CAD build for the part. Positions are in the model's coordinates, mm. Face numbers are marked on the shaded views. Round coordinates to 2 decimals unless told otherwise and drop trailing zeros. Write each loop counter-clockwise with the first axis right and the second up, starting at its lowest first coordinate (ties: lowest second). Pieces come first, ordered by that corner, then holes. Notation, with made-up numbers: (43.25, 20) -> (60.25, 20) arc R18 ccw to (60.25, 34) -> close; hole circle Ø7 at (10.5, -4.75). An arc over 180 degrees is marked (long way). Put each result on its own line as item: value. Start each with the question number.
1. Saw through at D-D on y = 2.75. List the corners of the cut face in (x, z).
2. Pull direction Z, two halves, no side cores. Call the marked faces 1, 2 and 3: pulls with the +Z half, pulls with the -Z half, needs draft (parallel to the pull), parting line crosses it, or undercut.
3. Saw through at C-C on z = -6.5. List the corners of the cut face in (x, y), and give its area (3 significant figures).
4. Saw through at A-A on x = 11. List the corners of the cut face in (y, z).
5. Drill centre lines: line 1 (Z direction, x = -7.5, y = 3.5); line 2 (X direction, y = 2.5, z = 4); line 3 (Z direction, x = 14.5, y = 1.5). Where is each one in solid material? Low to high. Write a range as from..to.
6. Flat gauge pins, fed straight in: P1, Ø1.9, axis at x = 27.81, y = 9.83, coming from the +Z side; P2, Ø8, axis at x = -13, y = 13.5, coming from the -Z side; P3, Ø5, axis at y = 7, z = -2.5, coming from the +X side; P4, Ø6, axis at x = -3, z = -7.5, coming from the +Y side. Where does each tip first touch, or does it go through?
7. Saw through at B-B on z = 3.5. List the corners of the cut face in (x, y).
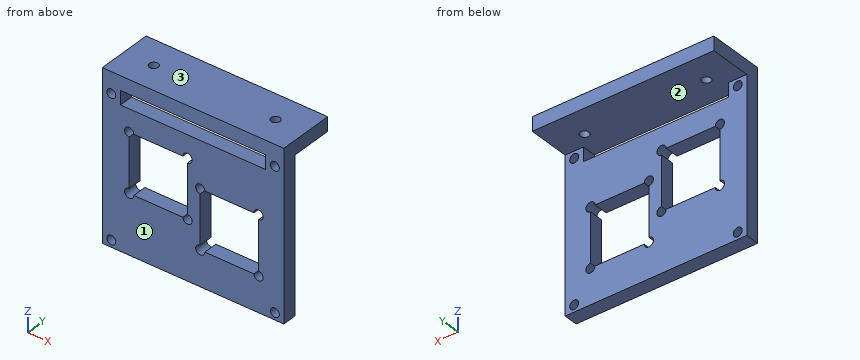
from build123d import *

# Parameters (mm, degrees)
SKETCH_1_R          = 1.6
EXTRUDE_1_DEPTH     = 5
SKETCH_2_R          = 1.65
SKETCH_2_W          = 20.88
SKETCH_2_H          = 20.88
CUT_EXTRUDE_1_DEPTH = 5
SKETCH_4_W          = 65
SKETCH_4_H          = 5
EXTRUDE_2_DEPTH     = 5
SKETCH_5_W          = 65
SKETCH_5_H          = 5
EXTRUDE_3_DEPTH     = 15
SKETCH_6_R          = 1.6
CUT_EXTRUDE_2_DEPTH = 15


with BuildPart() as part:
    # 草图1 → 凸台-拉伸1 (new body)
    with BuildSketch(Plane(origin=(0, 0, 0), x_dir=(1, 0, 0), z_dir=(0, 1, 0))):
        Polygon((-19.989784722, -25.876557595), (32.010215278, -25.876557595), (32.010215278, -30.876557595), (38.510215278, -30.876557595), (38.510215278, 24.123442405), (-26.489784722, 24.123442405), (-26.489784722, -30.876557595), (-19.989784722, -30.876557595), align=None)
        with Locations(Location((-23.259784722, 21.623442405, 0), (0, 0, 270))):
            Circle(SKETCH_1_R, mode=Mode.SUBTRACT)
        with Locations(Location((-23.259784722, -28.376557595, 0), (0, 0, 270))):
            Circle(SKETCH_1_R, mode=Mode.SUBTRACT)
        with Locations(Location((35.280215278, -28.376557595, 0), (0, 0, 270))):
            Circle(SKETCH_1_R, mode=Mode.SUBTRACT)
        with Locations(Location((35.280215278, 21.623442405, 0), (0, 0, 270))):
            Circle(SKETCH_1_R, mode=Mode.SUBTRACT)
    extrude(amount=EXTRUDE_1_DEPTH)

    # 草图2 → 切除-拉伸1 (cut)
    with BuildSketch(Plane(origin=(0, 5, 0), x_dir=(1, 0, 0), z_dir=(0, 1, 0))):
        with BuildLine():
            ThreePointArc((5.678835194, 2.978753935), (4.028835194, 4.628753935), (2.378835194, 2.978753935))
            Line((2.378835194, 2.978753935), (4.028835194, 2.978753935))
            Line((4.028835194, 2.978753935), (4.028835194, 1.328753935))
            ThreePointArc((4.028835194, 1.328753935), (5.195561383, 1.812027746), (5.678835194, 2.978753935))
        make_face()
        with BuildLine():
            Line((4.028835194, 2.978753935), (2.378835194, 2.978753935))
            ThreePointArc((2.378835194, 2.978753935), (2.862109005, 1.812027746), (4.028835194, 1.328753935))
            Line((4.028835194, 1.328753935), (4.028835194, 2.978753935))
        make_face()
        with Locations((-16.851164806, -17.901246065)):
            Circle(SKETCH_2_R)
        with Locations((4.028835194, -17.901246065)):
            Circle(SKETCH_2_R)
        with Locations((4.028835194, 2.978753935)):
            Circle(SKETCH_2_R)
        with Locations((-16.851164806, 2.978753935)):
            Circle(SKETCH_2_R)
        with Locations((-6.411164806, -7.461246065)):
            Rectangle(SKETCH_2_W, SKETCH_2_H)
        with BuildLine():
            ThreePointArc((5.678835194, -17.901246065), (5.195561383, -16.734519876), (4.028835194, -16.251246065))
            Line((4.028835194, -16.251246065), (4.028835194, -17.901246065))
            Line((4.028835194, -17.901246065), (2.378835194, -17.901246065))
            ThreePointArc((2.378835194, -17.901246065), (4.028835194, -19.551246065), (5.678835194, -17.901246065))
        make_face()
        with BuildLine():
            Line((4.028835194, -17.901246065), (4.028835194, -16.251246065))
            ThreePointArc((4.028835194, -16.251246065), (2.862109005, -16.734519876), (2.378835194, -17.901246065))
            Line((2.378835194, -17.901246065), (4.028835194, -17.901246065))
        make_face()
        with BuildLine():
            ThreePointArc((-15.201164806, -17.901246065), (-15.684438617, -16.734519876), (-16.851164806, -16.251246065))
            Line((-16.851164806, -16.251246065), (-16.851164806, -17.901246065))
            Line((-16.851164806, -17.901246065), (-15.201164806, -17.901246065))
        make_face()
        with BuildLine():
            Line((-16.851164806, -17.901246065), (-16.851164806, -16.251246065))
            ThreePointArc((-16.851164806, -16.251246065), (-18.017890995, -19.067972254), (-15.201164806, -17.901246065))
            Line((-15.201164806, -17.901246065), (-16.851164806, -17.901246065))
        make_face()
        with BuildLine():
            ThreePointArc((10.220215278, -9.316557595), (9.736941467, -8.149831407), (8.570215278, -7.666557595))
            Line((8.570215278, -7.666557595), (8.570215278, -9.316557595))
            Line((8.570215278, -9.316557595), (10.220215278, -9.316557595))
        make_face()
        with BuildLine():
            Line((8.570215278, -9.316557595), (8.570215278, -7.666557595))
            ThreePointArc((8.570215278, -7.666557595), (7.403489089, -10.483283784), (10.220215278, -9.316557595))
            Line((10.220215278, -9.316557595), (8.570215278, -9.316557595))
        make_face()
        with Locations((8.570215278, -9.316557595)):
            Circle(SKETCH_2_R)
        with Locations((29.450215278, -9.316557595)):
            Circle(SKETCH_2_R)
        with Locations((29.450215278, 11.563442405)):
            Circle(SKETCH_2_R)
        with Locations((8.570215278, 11.563442405)):
            Circle(SKETCH_2_R)
        with Locations((19.010215278, 1.123442405)):
            Rectangle(SKETCH_2_W, SKETCH_2_H)
        with BuildLine():
            ThreePointArc((31.100215278, 11.563442405), (29.450215278, 13.213442405), (27.800215278, 11.563442405))
            Line((27.800215278, 11.563442405), (29.450215278, 11.563442405))
            Line((29.450215278, 11.563442405), (29.450215278, 9.913442405))
            ThreePointArc((29.450215278, 9.913442405), (30.616941467, 10.396716216), (31.100215278, 11.563442405))
        make_face()
        with BuildLine():
            Line((29.450215278, 11.563442405), (27.800215278, 11.563442405))
            ThreePointArc((27.800215278, 11.563442405), (28.283489089, 10.396716216), (29.450215278, 9.913442405))
            Line((29.450215278, 9.913442405), (29.450215278, 11.563442405))
        make_face()
        with BuildLine():
            ThreePointArc((31.100215278, -9.316557595), (30.616941467, -8.149831407), (29.450215278, -7.666557595))
            Line((29.450215278, -7.666557595), (29.450215278, -9.316557595))
            Line((29.450215278, -9.316557595), (27.800215278, -9.316557595))
            ThreePointArc((27.800215278, -9.316557595), (29.450215278, -10.966557595), (31.100215278, -9.316557595))
        make_face()
        with BuildLine():
            Line((29.450215278, -9.316557595), (29.450215278, -7.666557595))
            ThreePointArc((29.450215278, -7.666557595), (28.283489089, -8.149831407), (27.800215278, -9.316557595))
            Line((27.800215278, -9.316557595), (29.450215278, -9.316557595))
        make_face()
    extrude(amount=-CUT_EXTRUDE_1_DEPTH, mode=Mode.SUBTRACT)

    # 草图4 → 凸台-拉伸2 (add)
    with BuildSketch(Plane.XY.offset(30.876557595)):
        with Locations((6.010215278, 2.5)):
            Rectangle(SKETCH_4_W, SKETCH_4_H)
    extrude(amount=EXTRUDE_2_DEPTH)

    # 草图5 → 凸台-拉伸3 (add)
    with BuildSketch(Plane(origin=(0, 5, 0), x_dir=(1, 0, 0), z_dir=(0, 1, 0))):
        with Locations((6.010215278, -33.376557595)):
            Rectangle(SKETCH_5_W, SKETCH_5_H)
    extrude(amount=EXTRUDE_3_DEPTH)

    # 草图6 → 切除-拉伸2 (cut)
    with BuildSketch(Plane(origin=(0, 0, 30.876557595), x_dir=(-1, 0, 0), z_dir=(0, 0, -1))):
        with Locations((-27.810215278, 9.832763387)):
            Circle(SKETCH_6_R)
        with Locations((15.789784722, 9.832763387)):
            Circle(SKETCH_6_R)
    extrude(amount=-CUT_EXTRUDE_2_DEPTH, mode=Mode.SUBTRACT)


solid = part.part
Return value:
1. outline: (-26.49, -24.12) -> (38.51, -24.12) -> (38.51, 35.88) -> (-26.49, 35.88) -> close; hole circle Ø3.2 at (-23.26, -21.62); hole circle Ø3.2 at (-23.26, 28.38); hole (-19.99, 25.88) -> (32.01, 25.88) -> (32.01, 30.88) -> (-19.99, 30.88) -> close; hole (-16.85, -1.33) arc R1.65 ccw (long way) to (-15.2, -2.98) -> (2.38, -2.98) arc R1.65 ccw (long way) to (4.03, -1.33) -> (4.03, 16.25) arc R1.65 ccw (long way) to (2.38, 17.9) -> (-15.2, 17.9) arc R1.65 ccw (long way) to (-16.85, 16.25) -> close; hole (8.57, -9.91) arc R1.65 ccw (long way) to (10.22, -11.56) -> (27.8, -11.56) arc R1.65 ccw (long way) to (29.45, -9.91) -> (29.45, 7.67) arc R1.65 ccw (long way) to (27.8, 9.32) -> (10.22, 9.32) arc R1.65 ccw (long way) to (8.57, 7.67) -> close; hole circle Ø3.2 at (35.28, -21.62); hole circle Ø3.2 at (35.28, 28.38)
2. face 1: needs draft
2. face 2: undercut
2. face 3: pulls with the +Z half
3. outline: (-26.49, 0) -> (8.57, 0) -> (8.57, 5) -> (-26.49, 5) -> close; (29.45, 0) -> (38.51, 0) -> (38.51, 5) -> (29.45, 5) -> close
3. area: 221 mm^2
4. outline: (0, -24.12) -> (5, -24.12) -> (5, -11.56) -> (0, -11.56) -> close; (0, 9.32) -> (5, 9.32) -> (5, 25.88) -> (0, 25.88) -> close; (0, 30.88) -> (20, 30.88) -> (20, 35.88) -> (0, 35.88) -> close
5. line 1: z = -24.12..-2.98, 17.9..25.88, 30.88..35.88
5. line 2: x = -26.49..-16.85, 4.03..8.57, 29.45..38.51
5. line 3: z = -24.12..-11.56, 9.32..25.88, 30.88..35.88
6. P1: passes through
6. P2: stops at z = 30.88
6. P3: stops at x = 38.51
6. P4: stops at y = 5
7. outline: (-26.49, 0) -> (-16.85, 0) -> (-16.85, 5) -> (-26.49, 5) -> close; (4.03, 0) -> (8.57, 0) -> (8.57, 5) -> (4.03, 5) -> close; (29.45, 0) -> (38.51, 0) -> (38.51, 5) -> (29.45, 5) -> close
